Geometry check sheet. Reference: the model listing, model coordinates, mm. Face numbers are marked on the shaded views. A direction names the side the tool comes from. Coordinates: 2 decimals unless noted, no trailing zeros. Loops run counter-clockwise (first coordinate to the right, second up) from the corner with the lowest first, then second, coordinate; pieces in that order, holes last.
from build123d import *

# Parameters (mm, degrees)
F0_W     = 30
F0_H     = 10
F1_DEPTH = 4
F2_W     = 34
F2_H     = 10
F3_DEPTH = 2
F4_W     = 30
F4_H     = 10
F5_DEPTH = 1.5
F6_W     = 30
F6_H     = 10
F7_DEPTH = 0.5


with BuildPart() as f1:
    # F0 (on Top) → F1 (new body)
    with BuildSketch(Plane.XY):
        Rectangle(F0_W, F0_H)
    extrude(amount=F1_DEPTH)

    # F2 (on face) → F3 (join)
    with BuildSketch(Plane.XY.offset(4)):
        Rectangle(F2_W, F2_H)
    extrude(amount=F3_DEPTH)

    # F4 (on face) → F5 (join)
    with BuildSketch(Plane.XY.offset(6)):
        Rectangle(F4_W, F4_H)
    extrude(amount=F5_DEPTH)

    # F6 (on face) → F7 (join)
    with BuildSketch(Plane.XY.offset(7.5)):
        Rectangle(F6_W, F6_H)
    extrude(amount=F7_DEPTH)


solid = f1.part
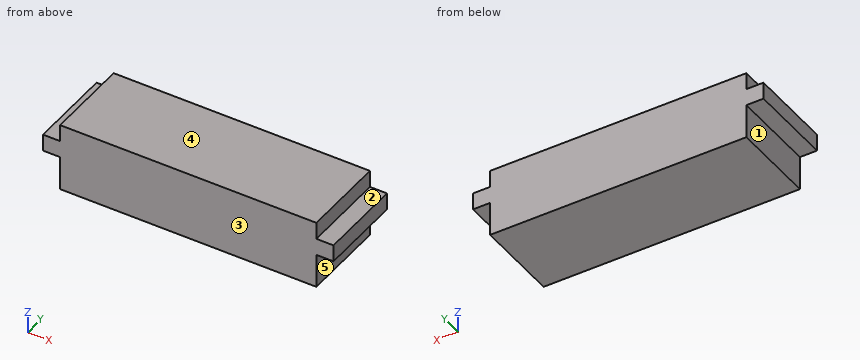
(1) Sectioned sample at A-A on y = 1.75. Record the cut outline in (x, z), and give its area (3 significant figures).
Findings:
outline: (-17, 4) - (-15, 4) - (-15, 0) - (15, 0) - (15, 4) - (17, 4) - (17, 6) - (15, 6) - (15, 8) - (-15, 8) - (-15, 6) - (-17, 6) - close
area: 248 mm2
(2) Sectioned sample at B-B on z = 1.75. Record the cut outline in (x, y), and give its area (3 significant figures).
Findings:
outline: (-15, -5) - (15, -5) - (15, 5) - (-15, 5) - close
area: 300 mm2
(3) Scan line: L1, parallel to X at y = -3, z = 0.5. Record every from-to range of solid material in increasing order.
Findings:
L1: x = -15 to 15
(4) Access from +Z, -Z, +X, -X, +Y, -Y to the whole of each face (thin tool, end or side, straight path). Record for the marked faces 1, 2, 3, 4 and 5.
Findings:
face 1: -Z, -X, +Y, -Y
face 2: +Z, +X, +Y, -Y
face 3: +Z, -Z, +X, -X, -Y
face 4: +Z, +X, -X, +Y, -Y
face 5: -Z, +X, +Y, -Y
(5) Gauge pin test, flat ends, axial feed: pin 1 Ø3 at (y, z) = (0, 2) entering from -X; pin 2 Ø0.6 at (x, y) = (-16, -1.5) entering from -Z; pin 3 Ø1.6 at (x, y) = (-16, 2) entering from +Z. Record the tip position at first contact, or that the pin passes through.
Findings:
pin 1: stops at x = -15
pin 2: stops at z = 4
pin 3: stops at z = 6
